Autodesk Inventor part; units mm, degrees
ref_plane "YZ Plane" through (0, 0, 0) normal (1, 0, 0) x (0, 1, 0)
ref_plane "XZ Plane" through (0, 0, 0) normal (0, 1, 0) x (-1, 0, 0)
ref_plane "XY Plane" through (0, 0, 0) normal (0, 0, 1) x (1, 0, 0)
sketch "Panel" plane through (0, 0, 0) normal (0, 0, 1) x (1, 0, 0)
  line L0 (-187.5, 125) -> (187.5, 125)
  line L1 (187.5, 125) -> (187.5, -125)
  line L2 (187.5, -125) -> (-187.5, -125)
  line L3 (-187.5, -125) -> (-187.5, 125)
  point P0 (0, 0)
  point P1 (-187.5, 0)
  point P2 (0, 125)
  dimension "d0" = 250
  dimension "d3" = 375
sketch "JoystickMount" plane through (0, 0, 0) normal (0, 0, 1) x (1, 0, 0)
  line L0 (-131.125, 55.25) -> (-131.125, 14.75) construction
  line L1 (-131.125, 14.75) -> (-46.125, 14.75) construction
  point P0 (0, 0)
  point P1 (-88.625, 35)
  point P2 (-46.125, 55.25)
  point P3 (-131.125, 35)
  point P4 (-88.625, 14.75)
  dimension "d4" = 40.5
  dimension "d6" = 85
  dimension "d19" = 35
  dimension "d45" = 88.625
sketch "ButtonMounts" plane through (0, 0, 0) normal (0, 0, 1) x (1, 0, 0)
  point P0 (0, 0)
  point P1 (6.375, 56)
  point P2 (6.375, 17)
  point P3 (37.625, 74)
  point P4 (37.625, 35)
  point P5 (73.625, 74)
  point P6 (73.625, 35)
  point P7 (108.625, 65)
  point P8 (108.625, 26)
  point P9 (-88.625, 35)
  dimension "d7" = 39
  dimension "d9" = 39
  dimension "d10" = 39
  dimension "d11" = 39
  dimension "d12" = 31.25
  dimension "d13" = 36
  dimension "d14" = 35
  dimension "d15" = 18
  dimension "d16" = 9
  dimension "d17" = 95
extrude "PanelExtrusion" add sketch "Panel" against normal blind 3
hole "JoystickScrews" at (-46.125, 14.75, 0) at (-46.125, 55.25, 0) at (-131.125, 55.25, 0) at (-131.125, 14.75, 0) direction (0, 0, -1) diameter 4.5 end through all countersink diameter 9.4 countersink angle 90
hole "JoystickShaft" at (-88.625, 35, 0) direction (0, 0, -1) diameter 24 end through all
hole "ButtonHoles" at (108.625, 26, 0) at (73.625, 35, 0) at (73.625, 74, 0) at (108.625, 65, 0) at (37.625, 74, 0) at (37.625, 35, 0) at (6.375, 56, 0) at (6.375, 17, 0) direction (0, 0, -1) diameter 30 end through all
fillet "PanelCornerFillets" radius 2 4 edges at (187.5, 125, -1.5) (187.5, -125, -1.5) (-187.5, 125, -1.5) (-187.5, -125, -1.5)
ref_plane "BottomPanelWorkPlane" through (187.5, -125, -3) normal (0, -0.1736, -0.9848) x (-1, 0, 0)
sketch "ProjectedEdgesBase" plane through (187.5, -125, -3) normal (0, -0.1736, -0.9848) x (-1, 0, 0)
  line L0 (0, 244.2323) -> (0, 1.9696)
  line L1 (373, 246.2019) -> (2, 246.2019)
  line L2 (375, 1.9696) -> (375, 244.2323)
  line L3 (2, -0.5209) -> (373, -0.5209)
  line L4 (375, 246.2019) -> (0, 246.2019)
  line L5 (0, 246.2019) -> (0, -0.5209)
  line L6 (0, -0.5209) -> (375, -0.5209)
  line L7 (375, -0.5209) -> (375, 246.2019)
  point P0 (187.5, 122.58)
  point P1 (187.5, 246.2019)
  point P2 (187.5, 246.2019)
  point P3 (187.5, -0.5209)
  point P4 (187.5, -0.5209)
  point P5 (375, 122.8405)
  point P6 (375, 123.101)
  point P7 (0, 122.8405)
  point P8 (0, 123.101)
properties part number "Panel_top_2"
Could you check a few things on this model? Use its own coordinates, in mm. Give positions to 0.01 mm unless a question says otherwise; leave off trailing zeros. Order: outer loops, then holes, each group sorted by start corner. A loop starts at its lowest first (then second) coordinate and runs counter-clockwise, first axis right, second up.
Item 1: If we section it at C-C, the plane z = -1.85: Count the separate pieces of the cut face and the enclosed holes in it, plus the area to 3 significant figures.
Item 2: If we section it at A-A, the plane x = 68.5: Write out the boundary of the cut face in (y, z), plus the area to 3 significant figures.
Item 3: If we section it at B-B, the plane y = 65: Write out the boundary of the cut face in (x, z) (3 decimals), plus the area to 3 significant figures.
Item 4: I'm going to push flat-ended pins straight in: pin 1 (4 mm diameter, centred on x = -131.125, y = 55.25, fed in from +Z); pin 2 (7 mm diameter, centred on x = -46.125, y = 55.25, fed in from +Z); pin 3 (7 mm diameter, centred on x = -131.125, y = 14.75, fed in from -Z); pin 4 (6 mm diameter, centred on x = -46.125, y = 14.75, fed in from +Z). Where does each tip first touch, or does it pass through?
Item 5: I need wall thicknesses on line 1 (X direction, y = 35, z = -1.4) (3 decimals); line 2 (X direction, y = 36.5, z = -2.4); line 3 (X direction, y = 25.5, z = -0.3). Which ranges of each line are inside material? Lowest first, please.
Values:
1. separate pieces: 1
1. enclosed holes: 13
1. area: 87,500 mm2
2. outline: (-125, -3) - (20.9, -3) - (20.9, 0) - (-125, 0) - close; (49.1, -3) - (59.9, -3) - (59.9, 0) - (49.1, 0) - close; (88.1, -3) - (125, -3) - (125, 0) - (88.1, 0) - close
2. area: 581 mm2
3. outline: (-187.5, -3) - (-5.625, -3) - (-5.625, 0) - (-187.5, 0) - close; (18.375, -3) - (25.625, -3) - (25.625, 0) - (18.375, 0) - close; (49.625, -3) - (61.625, -3) - (61.625, 0) - (49.625, 0) - close; (85.625, -3) - (93.625, -3) - (93.625, 0) - (85.625, 0) - close; (123.625, -3) - (187.5, -3) - (187.5, 0) - (123.625, 0) - close
3. area: 819 mm2
4. pin 1: passes through
4. pin 2: stops at z = -1.2
4. pin 3: stops at z = -3
4. pin 4: stops at z = -1.7
5. line 1: x = -187.5 to -100.625, -76.625 to 22.625, 52.625 to 58.625, 88.625 to 96.625, 120.625 to 187.5
5. line 2: x = -187.5 to -100.53, -76.72 to 22.7, 52.55 to 58.7, 88.55 to 97.91, 119.34 to 187.5
5. line 3: x = -187.5 to -95.96, -81.29 to -5.98, 18.73 to 26.02, 49.23 to 62.02, 85.23 to 93.63, 123.62 to 187.5
